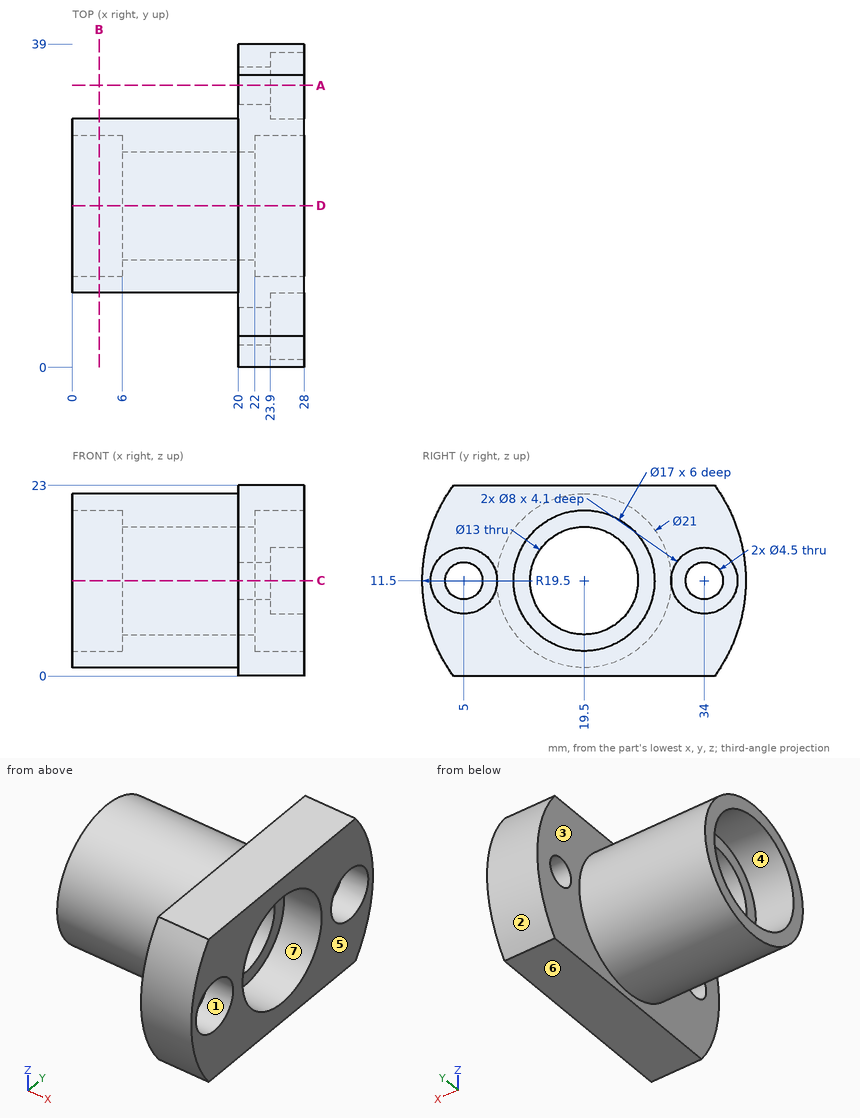
Print and shaded views of the part. All mm, measured from the part's lowest x, y and z. A direction names the side the tool comes from. Round coordinates to 2 decimals unless told otherwise and drop trailing zeros. Write each loop counter-clockwise with the first axis right and the second up, starting at its lowest first coordinate (ties: lowest second). Pieces come first, ordered by that corner, then holes. Notation, with made-up numbers: (45, 23) -> (85, 23) arc R20 cw to (85, 55) -> close; hole circle Ø3 at (5, 5.5). An arc over 180 degrees is marked (long way). Return JSON: item names as keys, results as strings. Group by question number.
Q1. Saw through at A-A on y = 34. Write the cut outline in (x, z).
Q2. Which spindle directions (+Z, -Z, +X, -X, +Y, -Y) get a long thin tool onto all of the face, cutting with end or side? Do the marked faces 1, 2 and 3. Say none if no direction does.
Q3. Saw through at C-C on z = 11.5. State how many separate pieces and enclosed holes the cut face has, plus the area to 3 significant figures.
Q4. Saw through at B-B on x = 3.25. Write the cut outline in (y, z).
Q5. Saw through at D-D on y = 19.5. Write the cut outline in (x, z).
Q6. Probe L1, parallel to Y at x = 22.15, z = 11.5; L2, parallel to Y at x = 4.25, z = 11.5; L3, parallel to Y at x = 25, z = 14.5. List the from-to ranges inside material, lowest first. Write a range as [from, to].
Q7. Pin check, flat tips, straight feed: pin 1 (5 mm diameter, centred on x = 14, y = 33, fed in from +Z); pin 2 (4 mm diameter, centred on y = 27.5, z = 10.5, fed in from +X); pin 3 (2 mm diameter, centred on x = 14.5, z = 5, fed in from +Y); pin 4 (5 mm diameter, centred on y = 5, z = 11.5, fed in from -X). Stop position of each tip, or through.
Q8. Mould opens along Z. For the marked faces 4, 5, 6 and 7 say: pulls with the +Z half, pulls with the -Z half, needs draft (parallel to the pull), parting line crosses it, or undercut.
Answer:
{
 "1": {"outline": "(20, 0) -> (28, 0) -> (28, 7.5) -> (23.9, 7.5) -> (23.9, 9.25) -> (20, 9.25) -> close; (20, 13.75) -> (23.9, 13.75) -> (23.9, 15.5) -> (28, 15.5) -> (28, 23) -> (20, 23) -> close"},
 "2": {"face 1": "+X", "face 2": "+X, -X, +Y", "face 3": "-X"},
 "3": {"separate pieces": "4", "enclosed holes": "0", "area": "219 mm2"},
 "4": {"outline": "circle Ø21 at (19.5, 11.5); hole circle Ø17 at (19.5, 11.5)"},
 "5": {"outline": "(0, 1) -> (20, 1) -> (20, 0) -> (28, 0) -> (28, 3) -> (22, 3) -> (22, 5) -> (6, 5) -> (6, 3) -> (0, 3) -> close; (0, 20) -> (6, 20) -> (6, 18) -> (22, 18) -> (22, 20) -> (28, 20) -> (28, 23) -> (20, 23) -> (20, 22) -> (0, 22) -> close"},
 "6": {"L1": "[0, 2.75], [7.25, 11], [28, 31.75], [36.25, 39]", "L2": "[9, 11], [28, 30]", "L3": "[0.23, 2.35], [7.65, 11.55], [27.45, 31.35], [36.65, 38.77]"},
 "7": {"pin 1": "through", "pin 2": "x = 28", "pin 3": "y = 28.44", "pin 4": "x = 20"},
 "8": {"face 4": "undercut", "face 5": "needs draft", "face 6": "pulls with the -Z half", "face 7": "undercut"}
}
